from build123d import *

# Parameters (mm, degrees)
BOSS_EXTRUDE1_DEPTH = 3.175
SKETCH2_R           = 3.4925
CUT_EXTRUDE2_DEPTH  = 3.175
LPATTERN5_COUNT     = 3
LPATTERN5_PITCH     = 22.86
SKETCH7_R           = 3.4925
CUT_EXTRUDE3_DEPTH  = 3.175
LPATTERN6_COUNT     = 2
LPATTERN6_PITCH     = 22.86
SKETCH8_R           = 3.4925
CUT_EXTRUDE4_DEPTH  = 85.115331985
FILLET3_R           = 12.7
FILLET4_R           = 3.175


with BuildPart() as part:
    # Sketch1 → Boss-Extrude1 (new body)
    with BuildSketch(Plane(origin=(0, 0, 0), x_dir=(1, 0, 0), z_dir=(0, 1, 0))):
        Polygon((-17.960512242, 17.960512242), (0, 35.921024484), (17.960512242, 17.960512242), (50.289434278, -14.368409794), (32.328922036, -32.328922036), (0, 0), (-31.430896424, -31.430896424), (-49.391408666, -13.470384182), align=None)
    extrude(amount=BOSS_EXTRUDE1_DEPTH)

    # Sketch2 → Cut-Extrude2 (cut)
    with BuildSketch(Plane(origin=(0, 3.175, 0), x_dir=(1, 0, 0), z_dir=(0, 1, 0))):
        with Locations(Location((-32.328922036, -14.368409794, 0), (0, 0, 270))):
            Circle(SKETCH2_R)
    cut_extrude2 = extrude(amount=-CUT_EXTRUDE2_DEPTH, mode=Mode.SUBTRACT)

    # LPattern5: Cut-Extrude2 ×3
    with Locations(*[Vector(0.7071067811865467, 0, -0.7071067811865485) * (i * LPATTERN5_PITCH) for i in range(1, LPATTERN5_COUNT)]):
        add(cut_extrude2, mode=Mode.SUBTRACT)

    # Sketch7 → Cut-Extrude3 (cut)
    with BuildSketch(Plane(origin=(0, 3.175, 0), x_dir=(1, 0, 0), z_dir=(0, 1, 0))):
        with Locations(Location((33.226947648, -15.266435406, 0), (0, 0, 270))):
            Circle(SKETCH7_R)
    cut_extrude3 = extrude(amount=-CUT_EXTRUDE3_DEPTH, mode=Mode.SUBTRACT)

    # LPattern6: Cut-Extrude3 ×2
    with Locations(*[Vector(-0.7071067811865457, 0, -0.7071067811865493) * (i * LPATTERN6_PITCH) for i in range(1, LPATTERN6_COUNT)]):
        add(cut_extrude3, mode=Mode.SUBTRACT)

    # Mirror2: part across plane


with BuildPart() as part_1:
    add(part.part)
    add(part.part.mirror(Plane(origin=(8.980256121, 0, -8.980256121), x_dir=(0.7071067811865464, 0, 0.7071067811865487), z_dir=(-0.7071067811865489, 0, 0.7071067811865462))))

    # Sketch8 → Cut-Extrude4 (cut, through all)
    # profile 1 of 3: a face of its own
    with BuildSketch(Plane(origin=(0, 3.175, 0), x_dir=(1, 0, 0), z_dir=(0, 1, 0))):
        Polygon((-15.266435406, -15.266435406), (-33.226947648, 2.694076836), (-49.391408666, -13.470384182), (-31.430896424, -31.430896424), align=None)
        with Locations((-32.328922036, -14.368409794)):
            Circle(SKETCH8_R, mode=Mode.SUBTRACT)
    # profile 2 of 3: a face of its own
    with BuildSketch(Plane(origin=(0, 3.175, 0), x_dir=(1, 0, 0), z_dir=(0, 1, 0))):
        Polygon((33.226947648, 33.226947648), (49.391408666, 49.391408666), (31.430896424, 67.351920908), (15.266435406, 51.18745989), align=None)
        with Locations((32.328922036, 50.289434278)):
            Circle(SKETCH8_R, mode=Mode.SUBTRACT)
    # profile 3 of 3: a face of its own
    with BuildSketch(Plane(origin=(0, 3.175, 0), x_dir=(1, 0, 0), z_dir=(0, 1, 0))):
        Polygon((50.289434278, -14.368409794), (34.12497326, 1.796051224), (16.164461018, -16.164461018), (32.328922036, -32.328922036), align=None)
        with Locations((33.226947648, -15.266435406)):
            Circle(SKETCH8_R, mode=Mode.SUBTRACT)
    extrude(amount=-CUT_EXTRUDE4_DEPTH, mode=Mode.SUBTRACT)

    # Fillet3
    fillet3_edges = [part_1.edges().sort_by_distance(p)[0] for p in [
        (0, 1.5875, 0),
        (17.960512242, 1.5875, -17.960512242),
    ]]
    fillet(fillet3_edges, radius=FILLET3_R)

    # Fillet4
    fillet4_edges = [part_1.edges().sort_by_distance(p)[0] for p in [
        (-33.226947648, 1.5875, -2.694076836),
        (-15.266435406, 1.5875, 15.266435406),
        (15.266435406, 1.5875, -51.18745989),
        (33.226947648, 1.5875, -33.226947648),
        (16.164461018, 1.5875, 16.164461018),
        (34.12497326, 1.5875, -1.796051224),
    ]]
    fillet(fillet4_edges, radius=FILLET4_R)


solid = part_1.part
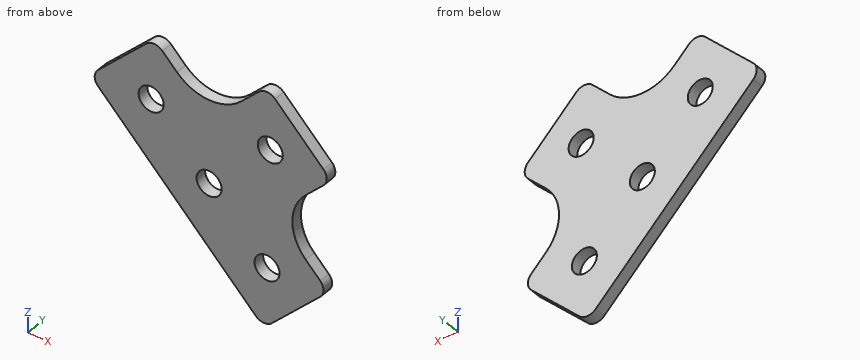
Build history of the part. All positions in model axes, mm. Round coordinates to 2 decimals unless told otherwise and drop trailing zeros. Order: outer loops, then holes, each group sorted by start corner. A loop starts at its lowest first (then second) coordinate and runs counter-clockwise, first axis right, second up. Notation, with made-up numbers: M 57.5,-21 L 94.5,-21 A30 ccw 94.5,15 Z; hole C 87,81 d5. An arc over 180 degrees is marked long. Use CSV: the item, a comma, the result in double quotes. Start each with the question number.
(1) Drill centre lines: probe 1 along X at (y, z) = (0.9, -35); probe 2 along X at (y, z) = (0.6, -0.5); probe 3 along Z at (x, y) = (-18.5, 0.25). Where is each one in solid material? Low to high.
(2) Cut at D-D on x = 0. List the corners of the cut face in (y, z) (3 decimals), then the cut area to 3 significant figures.
(3) Cut at B-B on z = -17. List the corners of the cut face in (x, y) (3 decimals), then the cut area to 3 significant figures.
(4) Cut at A-A on x = 15.5. List the corners of the cut face in (y, z) (3 decimals), then the cut area to 3 significant figures.
(5) Cut at C-C on y = 2.4. State how many separate pieces and enclosed holes the cut face has, then the cut area to 3 significant figures.
Findings:
1,probe 1,"x = -0.92 to 12.78, 19.55 to 31.37"
1,probe 2,"x = -31.03 to -19.41, -12.92 to 13.59, 20.53 to 32.53"
1,probe 3,"z = -17.42 to -4.39, 0.8 to 12.03"
2,outline,"M 0,-35.921 L 3.175,-35.921 L 3.175,-21.453 L 0,-21.453 Z; M 0,-14.468 L 3.175,-14.468 L 3.175,5.261 L 0,5.261 Z"
2,area,"109 mm^2"
3,outline,"M -18.921,0 L -3.358,0 L -3.358,3.175 L -18.921,3.175 Z; M 3.358,0 L 23.257,0 L 23.257,3.175 L 3.358,3.175 Z"
3,area,"113 mm^2"
4,outline,"M 0,-49.864 L 3.175,-49.864 L 3.175,-37.554 L 0,-37.554 Z; M 0,-30.696 L 3.175,-30.696 L 3.175,-4.022 L 0,-4.022 Z; M 0,2.225 L 3.175,2.225 L 3.175,14.779 L 0,14.779 Z"
4,area,"164 mm^2"
5,separate pieces,"1"
5,enclosed holes,"4"
5,area,"2,230 mm^2"
